Read the model definition and answer for the solid it produces. Units are mm, in the model's axes. A direction names the side the tool comes from. Coordinates: 2 decimals unless noted, no trailing zeros. Loops run counter-clockwise (first coordinate to the right, second up) from the corner with the lowest first, then second, coordinate; pieces in that order, holes last. Notation, with made-up numbers: (48.25, 50.25) -> (94.25, 50.25) arc R22 ccw to (94.25, 78.25) -> close; hole circle Ø6 at (43, 63). An arc over 180 degrees is marked (long way). Answer as a JSON object with one key per item and string values. Group by question number.
Q1. The part is cut by section C-C on y = 34. Write down the section's boundary in (x, z).
Q2. For faces 1 (the flat face through (0, 59, 8)), 2 (the flat face through (-9, 28.7, 8)), determine the directions among +Z, -Z, +X, -X, +Y, -Y from which every point of the face is accessible in a straight line to the end or side of a thin tool.
Q3. The part is cut by section D-D on z = 7.75. State how many separate pieces and enclosed holes the cut face has, and give its area (3 significant figures).
Q4. The part is cut by section B-B on x = -8.75. Write down the section's boundary in (y, z), and give its area (3 significant figures).
Q5. Straight lines are drawn through the part: line 1 along X through (y, z) = (25, 4.5); line 2 along X through (y, z) = (27, 1.25). For each, find the intervals that lie inside material, in ascending order. Write a range as [from, to].
Q6. Each of these flat-tipped pins is pushed along its axis until it touches: P1, Ø0.7, axis at x = -7.14, y = 47, coming from the -Z side; P2, Ø4, axis at x = -10.5, z = 6, coming from the +Y side; P3, Ø8, axis at x = -7.5, z = 4, coming from the +Y side; P4, Ø8, axis at y = 18.5, z = 6, coming from the -X side. Where does it stop, or does it pass through?
Q7. The part is cut by section A-A on y = 43. Write down the section's boundary in (x, z), and give its area (3 significant figures).
from build123d import *

# Parameters (mm, degrees)
ESQUISSE1_R        = 1.6
BOSS_EXTRU_1_DEPTH = 15


with BuildPart() as part:
    # Esquisse1 → Boss.-Extru.1 (new body)
    with BuildSketch(Plane.XY.offset(15)):
        with BuildLine():
            Line((0, 57), (0, 61.5))
            ThreePointArc((0, 61.5), (-14.418041681, 32.032323515), (-21.5, 0))
            Line((-21.5, 0), (0, 0))
            Line((0, 0), (0, 3))
            ThreePointArc((0, 3), (-2.977286407, 30), (0, 57))
        make_face()
        with Locations(Location((-17.168486885, 2.5, 0), (0, 0, 180))):
            Circle(ESQUISSE1_R, mode=Mode.SUBTRACT)
        with BuildLine():
            Line((-4.312692911, 41), (-9.295115102, 41))
            ThreePointArc((-9.295115102, 41), (-10.303844451, 40.696573922), (-9.629905592, 41.50614708))
            ThreePointArc((-9.629905592, 41.50614708), (-8.526904057, 44.016241784), (-7.373977837, 46.503800615))
            ThreePointArc((-7.373977837, 46.503800615), (-7.430000368, 47.465288022), (-6.586730771, 47))
            Line((-6.586730771, 47), (-3.520929736, 47))
            ThreePointArc((-3.520929736, 47), (-2.553456769, 47.358073068), (-3.054688564, 46.456415178))
            ThreePointArc((-3.054688564, 46.456415178), (-3.40258545, 44.004720773), (-3.702576558, 41.546704695))
            ThreePointArc((-3.702576558, 41.546704695), (-3.3956534, 40.590387992), (-4.312692911, 41))
        make_face(mode=Mode.SUBTRACT)
        with BuildLine():
            Line((-10.442809639, 38.2), (-4.583085107, 38.2))
            ThreePointArc((-4.583085107, 38.2), (-3.628372615, 38.572434959), (-4.078693111, 37.651894253))
            ThreePointArc((-4.078693111, 37.651894253), (-4.283108767, 34.702786262), (-4.418771813, 31.7497168))
            ThreePointArc((-4.418771813, 31.7497168), (-4.053800983, 30.804901148), (-4.986419458, 31.2))
            Line((-4.986419458, 31.2), (-13.004497683, 31.2))
            ThreePointArc((-13.004497683, 31.2), (-14.001308767, 30.879282281), (-13.378533522, 31.721091752))
            ThreePointArc((-13.378533522, 31.721091752), (-12.321188046, 34.717395466), (-11.194758267, 37.688417405))
            ThreePointArc((-11.194758267, 37.688417405), (-11.302186638, 38.654737147), (-10.442809639, 38.2))
        make_face(mode=Mode.SUBTRACT)
        with BuildLine():
            Line((-3.015101171, 50), (-5.099632839, 50))
            ThreePointArc((-5.099632839, 50), (-6.119039194, 49.7133684), (-5.398388017, 50.489260707))
            ThreePointArc((-5.398388017, 50.489260707), (-3.263933011, 54.463678409), (-1, 58.365793421))
            Line((-1, 58.365793421), (-1, 56.97280273))
            ThreePointArc((-1, 56.97280273), (-1.724659998, 53.765748342), (-2.365989319, 50.540996156))
            ThreePointArc((-2.365989319, 50.540996156), (-2.112973011, 49.577500581), (-3.015101171, 50))
        make_face(mode=Mode.SUBTRACT)
        with BuildLine():
            Line((-3.89894146, 10.4), (-18.215006404, 10.4))
            ThreePointArc((-18.215006404, 10.4), (-19.185396456, 10.045356229), (-18.672359875, 10.942140776))
            ThreePointArc((-18.672359875, 10.942140776), (-18.026202705, 14.411865345), (-17.291034109, 17.863826355))
            ThreePointArc((-17.291034109, 17.863826355), (-17.51134183, 18.830058701), (-16.618486885, 18.4))
            Line((-16.618486885, 18.4), (-4.723453535, 18.4))
            ThreePointArc((-4.723453535, 18.4), (-3.799031061, 18.802874436), (-4.133243311, 17.851471844))
            ThreePointArc((-4.133243311, 17.851471844), (-3.82459023, 14.393466491), (-3.421455125, 10.945198834))
            ThreePointArc((-3.421455125, 10.945198834), (-2.935188807, 10.037634519), (-3.89894146, 10.4))
        make_face(mode=Mode.SUBTRACT)
        with BuildLine():
            Line((-13.816577523, 28.7), (-5.036607306, 28.7))
            ThreePointArc((-5.036607306, 28.7), (-4.096135841, 29.087339689), (-4.491036271, 28.150017833))
            ThreePointArc((-4.491036271, 28.150017833), (-4.464411374, 24.698655463), (-4.343932147, 21.249293805))
            ThreePointArc((-4.343932147, 21.249293805), (-3.917431797, 20.321070157), (-4.866069695, 20.7))
            Line((-4.866069695, 20.7), (-16.067033334, 20.7))
            ThreePointArc((-16.067033334, 20.7), (-17.050709214, 20.361732013), (-16.483125083, 21.233449698))
            ThreePointArc((-16.483125083, 21.233449698), (-15.552375348, 24.717038741), (-14.53042622, 28.174972758))
            ThreePointArc((-14.53042622, 28.174972758), (-14.692448063, 29.143067028), (-13.816577523, 28.7))
        make_face(mode=Mode.SUBTRACT)
        with BuildLine():
            Line((-18.53749956, 8.4), (-3.612290325, 8.4))
            ThreePointArc((-3.612290325, 8.4), (-2.704133874, 8.817401433), (-2.978748665, 7.85638176))
            ThreePointArc((-2.978748665, 7.85638176), (-2.747523602, 6.426825008), (-2.5, 5))
            Line((-2.5, 5), (-19.566563167, 5))
            ThreePointArc((-19.566563167, 5), (-19.375761002, 6.429149671), (-19.169954701, 7.856215898))
            ThreePointArc((-19.169954701, 7.856215898), (-19.446072894, 8.81704336), (-18.53749956, 8.4))
        make_face(mode=Mode.SUBTRACT)
        with BuildLine():
            Line((-3.068400716, 0.9), (-12.868400716, 0.9))
            ThreePointArc((-12.868400716, 0.9), (-14.468400716, 2.5), (-12.868400716, 4.1))
            Line((-12.868400716, 4.1), (-3.068400716, 4.1))
            ThreePointArc((-3.068400716, 4.1), (-1.468400716, 2.5), (-3.068400716, 0.9))
        make_face(mode=Mode.SUBTRACT)
    extrude(amount=-BOSS_EXTRU_1_DEPTH)


solid = part.part
Final values:
{
 "1": {"outline": "(-13.71, 0) -> (-12.58, 0) -> (-12.58, 15) -> (-13.71, 15) -> close; (-4.32, 0) -> (-2.91, 0) -> (-2.91, 15) -> (-4.32, 15) -> close"},
 "2": {"face 1": "+Z, -Z, +X, +Y, -Y", "face 2": "+Z, -Z"},
 "3": {"separate pieces": "1", "enclosed holes": "8", "area": "301 mm2"},
 "4": {"outline": "(0, 0) -> (0.9, 0) -> (0.9, 15) -> (0, 15) -> close; (4.1, 0) -> (5, 0) -> (5, 15) -> (4.1, 15) -> close; (8.4, 0) -> (10.4, 0) -> (10.4, 15) -> (8.4, 15) -> close; (18.4, 0) -> (20.7, 0) -> (20.7, 15) -> (18.4, 15) -> close; (28.7, 0) -> (31.2, 0) -> (31.2, 15) -> (28.7, 15) -> close; (38.2, 0) -> (41, 0) -> (41, 15) -> (38.2, 15) -> close; (43.52, 0) -> (45.82, 0) -> (45.82, 15) -> (43.52, 15) -> close", "area": "205 mm2"},
 "5": {"line 1": "x = [-16.67, -15.47], [-4.47, -2.88]", "line 2": "x = [-16.07, -14.89], [-4.49, -2.94]"},
 "6": {"P1": "passes through", "P2": "stops at y = 46.34", "P3": "stops at y = 55.79", "P4": "stops at x = -19.28"},
 "7": {"outline": "(-10.05, 0) -> (-8.98, 0) -> (-8.98, 15) -> (-10.05, 15) -> close; (-3.53, 0) -> (-2.29, 0) -> (-2.29, 15) -> (-3.53, 15) -> close", "area": "34.6 mm2"}
}
